```python
from build123d import *

# Parameters (mm, degrees)
F0_W     = 520.7
F0_H     = 323.85
F1_DEPTH = 7.62
F3_R     = 88.9
F3_R_2   = 57.15
F4_DEPTH = 7.62
F5_W     = 85.19419
F5_H     = 25.4
F6_DEPTH = 38.1
F8_DEPTH = 85.19419


with BuildPart() as f1:
    # F0 (on Front) → F1 (new body)
    with BuildSketch(Plane.XZ):
        with Locations((260.35, 161.925)):
            Rectangle(F0_W, F0_H)
    extrude(amount=-F1_DEPTH)



with BuildPart() as f4:
    # F3 (on offset) → F4 (new body)
    with BuildSketch(Plane.XY.offset(-69.85)):
        with Locations((260.35, 25.4)):
            Circle(F3_R)
        with Locations((260.35, 25.4)):
            Circle(F3_R_2, mode=Mode.SUBTRACT)
    extrude(amount=F4_DEPTH)

    # F5 (on offset) → F6 (join)
    with BuildSketch(Plane.XY.offset(-69.85)):
        with Locations((260.35, 76.2)):
            Rectangle(F5_W, F5_H)
    extrude(amount=F6_DEPTH)


with BuildPart() as f1_1:
    add(f1.part)

    add(f4.part)  # F8 merges F4
    # F7 (on face) → F8 (join, through all)
    with BuildSketch(Plane.YZ.offset(302.947095)):
        Polygon((7.62, 31.75), (63.5, -31.75), (88.9, -31.75), (13.97, 107.95), (7.62, 107.95), align=None)
    extrude(amount=-F8_DEPTH)


solid = f1_1.part
```
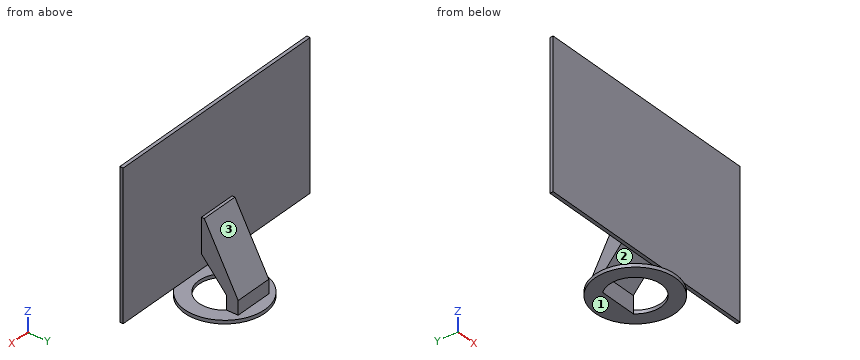
The listing builds one solid part. Answer for the finished solid, in the listing's coordinates (mm). Face numbers are marked on the shaded views. Coordinates: 2 decimals unless noted, no trailing zeros. Write each loop counter-clockwise with the first axis right and the second up, starting at its lowest first coordinate (ties: lowest second). Pieces come first, ordered by that corner, then holes. Notation, with made-up numbers: M 28,26 L 56,26 A28 ccw 56,47 Z; hole C -30.5,-7.75 d5. An arc over 180 degrees is marked long. Use a Markdown table: item, result. Add a question column.
1. For a pull along Y with two mould halves and no side action, classify the marked faces 1, 2 and 3 as +Y half, -Y half, draft (parallel to the pull), parting line (faces both ways), or undercut.
2. Section C-C (z = 54) is taken. Give the vertices of the cut face in (x, y), plus the area to 3 significant figures.
3. Straight lines are drawn through the part: line 1 along Y through (x, z) = (53, 56); line 2 along X through (y, z) = (25, -64); line 3 along Y through (x, z) = (260, -66). For each, find the intervals that lie inside material, in ascending order. Write a range as [from, to].
4. Given P1, Ø3, axis at x = 208.5, z = 65, coming from the +Y side; P2, Ø3, axis at x = 249, y = 9.5, coming from the +Z side; P3, Ø11.5, axis at x = 245.5, z = -60, coming from the -Y side, each flat-ended and moving along its own axis, determine where each tip first touches the part or whether it passes through.
5. Section A-A (x = 260.35) is taken. Give the vertices of the cut face in (y, z), plus the area to 3 significant figures.
6. Section B-B (y = 55.5) is taken. Give the vertices of the cut face in (x, z), plus the area to 3 significant figures.
7. Section D-D (y = -11) is taken. Give the vertices of the cut face in (x, z).
Data:
| question | item | result |
|---|---|---|
| 1 | face 1 | draft |
| 1 | face 2 | undercut |
| 1 | face 3 | +Y half |
| 2 | outline | M 0,0 L 520.7,0 L 520.7,7.62 L 302.95,7.62 L 302.95,42.91 L 217.75,42.91 L 217.75,7.62 L 0,7.62 Z |
| 2 | area | 6,970 mm2 |
| 3 | line 1 | y = [0, 7.62] |
| 3 | line 2 | x = [171.45, 203.2], [317.5, 349.25] |
| 3 | line 3 | y = [-63.5, -31.75], [63.5, 114.3] |
| 4 | P1 | stops at y = 7.62 |
| 4 | P2 | stops at z = 107.95 |
| 4 | P3 | stops at y = -62.99 |
| 5 | outline | M -63.5,-69.85 L -31.75,-69.85 L -31.75,-62.23 L -63.5,-62.23 Z; M 0,0 L 7.62,0 L 7.62,31.75 L 63.5,-31.75 L 63.5,-69.85 L 114.3,-69.85 L 114.3,-62.23 L 88.9,-62.23 L 88.9,-31.75 L 13.97,107.95 L 7.62,107.95 L 7.62,323.85 L 0,323.85 Z |
| 5 | area | 8,220 mm2 |
| 6 | outline | M 176.7,-69.85 L 211.77,-69.85 L 211.77,-62.23 L 176.7,-62.23 Z; M 217.75,-22.66 L 302.95,-22.66 L 302.95,30.52 L 217.75,30.52 Z; M 308.93,-69.85 L 344,-69.85 L 344,-62.23 L 308.93,-62.23 Z |
| 6 | area | 5,070 mm2 |
| 7 | outline | M 179.24,-69.85 L 216.29,-69.85 L 216.29,-62.23 L 179.24,-62.23 Z; M 304.41,-69.85 L 341.46,-69.85 L 341.46,-62.23 L 304.41,-62.23 Z |
